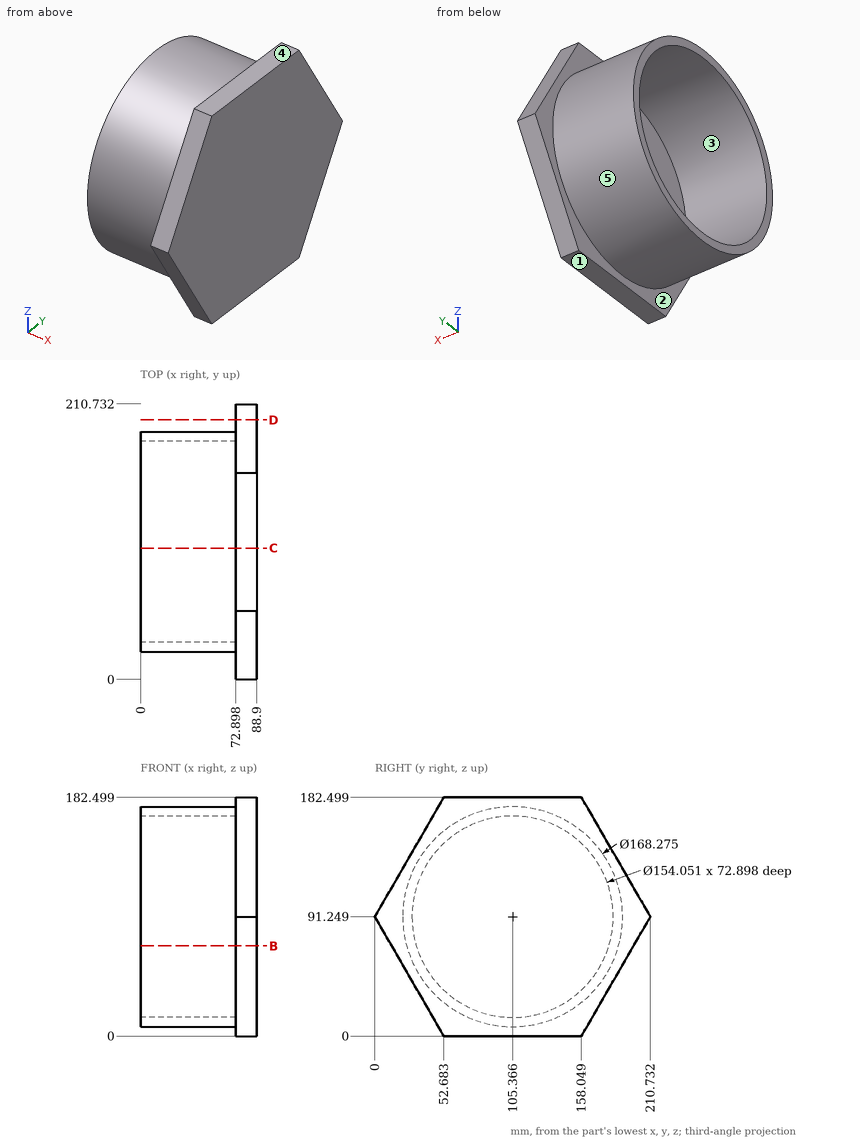
Input: dimensioned drawing with shaded views. Units: mm. Origin: part minimum x, y, z. A direction names the side the tool comes from. Coordinates: 2 decimals unless noted, no trailing zeros. Loops run counter-clockwise (first coordinate to the right, second up) from the corner with the lowest first, then second, coordinate; pieces in that order, holes last.
Q1. Set-up query: the marked faces 1 and 2. Return all of +Z, -Z, +X, -X, +Y, -Y with unobstructed straight access to the full face (end or side cutting, diameter ignored); none if empty.
Results are:
face 1: -Z, +X, -X, +Y, -Y
face 2: -X
Q2. Line query: line 1 along Y through (x, z) = (67.5, 92) (1 decimal); line 2 along Z through (x, y) = (46, 103) (1 decimal); line 3 along Y through (x, z) = (9, 47) (1 decimal). Output: solid intervals per line, ascending.
Results are:
line 1: y = 21.2 to 28.3, 182.4 to 189.5
line 2: z = 7.1 to 14.3, 168.2 to 175.4
line 3: y = 33.8 to 42.3, 168.4 to 176.9
Q3. Section C-C, the plane y = 100.5. Return the cut outline in (x, z), and give its area (3 significant figures).
Results are:
outline: (0, 7.25) - (72.9, 7.25) - (72.9, 0) - (88.9, 0) - (88.9, 182.5) - (72.9, 182.5) - (72.9, 175.25) - (0, 175.25) - (0, 168.12) - (72.9, 168.12) - (72.9, 14.38) - (0, 14.38) - close
area: 3,960 mm2
Q4. Section D-D, the plane y = 198.5. Return the cut outline in (x, z) (1 decimal), and give its area (3 significant figures).
Results are:
outline: (72.9, 70.1) - (88.9, 70.1) - (88.9, 112.4) - (72.9, 112.4) - close
area: 678 mm2
Q5. Contact query for flat-ended pins moving along their axis: pin 1 (10 mm diameter, centred on y = 80.5, z = 111.5, fed in from -X); pin 2 (1 mm diameter, centred on x = 13.5, y = 96, fed in from +Z); pin 3 (1 mm diameter, centred on x = 19, z = 71, fed in from +Y); pin 4 (2 mm diameter, centred on x = 80, y = 120, fed in from -Z). Output: stop coordinate, or through.
Results are:
pin 1: stops at x = 72.9
pin 2: stops at z = 174.92
pin 3: stops at y = 187.15
pin 4: stops at z = 0
Q6. Mould query, pull axis Z, two halves, no side actions, for the marked faces 3, 4 and 5. Classes: +Z half, -Z half, draft (parallel to the pull), parting line (faces both ways), or undercut.
Results are:
face 3: undercut
face 4: +Z half
face 5: parting line
Q7. Section B-B, the plane z = 69. Return the cut outline in (x, y) (1 decimal).
Results are:
outline: (0, 24.2) - (72.9, 24.2) - (72.9, 12.8) - (88.9, 12.8) - (88.9, 197.9) - (72.9, 197.9) - (72.9, 186.5) - (0, 186.5) - (0, 179.1) - (72.9, 179.1) - (72.9, 31.6) - (0, 31.6) - close
